```python
from build123d import *

# Parameters (mm, degrees)
F0_W     = 50
F0_H     = 50
F1_DEPTH = 25
F2_R     = 12.5410475497
F3_DEPTH = 25
F5_DEPTH = 25
F7_DEPTH = 50
F9_DEPTH = 25
F10_R    = 5


with BuildPart() as f1:
    # F0 (on Front) → F1 (new body)
    with BuildSketch(Plane.XZ):
        Rectangle(F0_W, F0_H)
    extrude(amount=F1_DEPTH)

    # F2 (on face) → F3 (cut)
    with BuildSketch(Plane.XZ.offset(25)):
        Circle(F2_R)
    extrude(amount=-F3_DEPTH, mode=Mode.SUBTRACT)

    # F4 (on face) → F5 (join)
    with BuildSketch(Plane.XZ.offset(25)):
        with BuildLine():
            Line((-8.8678597656, -8.8678597656), (-25, -25))
            Line((-25, -25), (25, -25))
            Line((25, -25), (25, 25))
            Line((25, 25), (8.8678597656, 8.8678597656))
            ThreePointArc((8.8678597656, 8.8678597656), (11.5864171474, 4.7992511218), (12.5410475497, 0))
            ThreePointArc((12.5410475497, 0), (4.7992511218, -11.5864171474), (-8.8678597656, -8.8678597656))
        make_face()
    extrude(amount=F5_DEPTH)

    # F6 (on face) → F7 (cut)
    with BuildSketch(Plane(origin=(0, 0, 0), x_dir=(0, -1, 0), z_dir=(-0.7071067812, 0, 0.7071067812))):
        Polygon((28.62248093, -26.3251687907), (35.0618112076, -33.3145719446), (44.3344770349, -31.2326499178), (47.1678125847, -22.1613247372), (40.7284823072, -15.1719215833), (31.4558164798, -17.2538436101), align=None)
        Polygon((27.4971282132, 24.391054001), (41.3385996573, 13.714221481), (43.6642721295, 31.0397036374), align=None)
    extrude(amount=-F7_DEPTH, mode=Mode.SUBTRACT)

    # F8 (on face) → F9 (join)
    with BuildSketch(Plane.XZ.offset(25)):
        Polygon((-20.9768815232, 21.2787960948), (-24.3413792657, 11.5523586689), (-16.1306745515, 5.3468967076), (-7.691682224, 11.2381477254), (-10.6868028491, 21.084603052), align=None)
    extrude(amount=F9_DEPTH)

    # F10
    f10_edges = [f1.edges().sort_by_distance(p)[0] for p in [
        (25, 0, 0),
        (0, 0, 25),
        (-25, 0, 0),
        (0, 0, -25),
    ]]
    fillet(f10_edges, radius=F10_R)


solid = f1.part
```
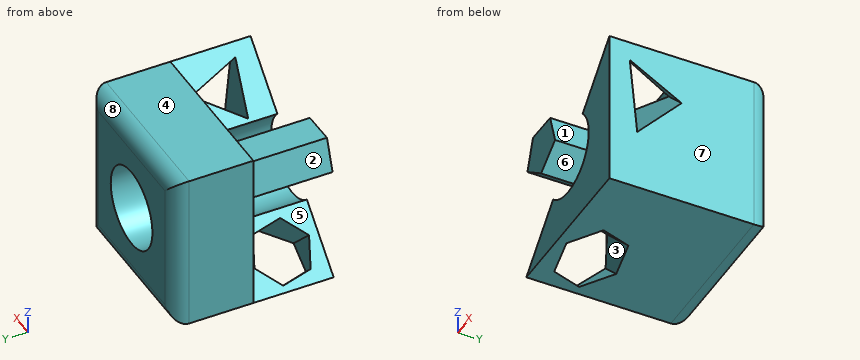
Check sheet for the modelled part. Datum: model origin and axes. Units: mm. Face numbers are marked on the shaded views. A direction names the side the tool comes from. Round coordinates to 2 decimals unless told otherwise and drop trailing zeros. Write each loop counter-clockwise with the first axis right and the second up, starting at its lowest first coordinate (ties: lowest second). Pieces come first, ordered by that corner, then holes. Notation, with made-up numbers: (47, 7.5) -> (90, 7.5) arc R9 ccw to (90, 15.5) -> close; hole circle Ø9 at (35.25, 22). An arc over 180 degrees is marked (long way). One line per question, with ' | ' between items. Start each with the question number.
1. Sectioned sample at C-C, the plane x = 10.5. Record the cut outline in (y, z).
2. Sectioned sample at D-D, the plane y = -39. Record the cut outline in (x, z), then the cut area to 3 significant figures.
3. Depth check by flat-ended pin: pin 1 (1.5 mm diameter, centred on y = -26.5, z = -15, fed in from -X). Enter the tip coordinate at first touch or a pass-through.
4. Release check for a two-part mould opening along Z. For the marked faces 6, 7 and 8 record: +Z half, -Z half, draft (parallel to the pull), parting line (faces both ways), or undercut.
5. Scan lines: line 1 along X through (y, z) = (-17.25, 0); line 2 along Y through (x, z) = (15, 5.5). Record each from-to range of solid material in increasing order. Write a range as from..to.
6. Set-up check for the marked faces 1, 2, 3, 4 and 5: record each of +Z, -Z, +X, -X, +Y, -Y from which the full face is reachable in a straight line by a thin tool's end or side.
7. Sectioned sample at A-A, the plane z = -10. Record the cut outline in (x, y), then the cut area to 3 significant figures.
8. Sectioned sample at B-B, the plane y = -20. Record the cut outline in (x, z), then the cut area to 3 significant figures.
Taken from the geometry:
1) outline: (-50, -25) -> (-5, -25) arc R5 ccw to (0, -20) -> (0, -6.86) -> (-50, -6.86) -> close; (-50, 6.86) -> (0, 6.86) -> (0, 20) arc R5 ccw to (-5, 25) -> (-25, 25) -> (-25, 10.5) -> (-39.87, 10.5) -> (-41.34, 8.89) -> (-41.49, 10.5) -> (-50, 10.5) -> close
2) outline: (-25, -25) -> (-20.86, -25) -> (-22.93, -22.93) -> close; (-24.34, 11.55) -> (-16.13, 5.35) -> (-7.69, 11.24) -> (-10.69, 21.08) -> (-20.98, 21.28) -> close; (-11, -11) -> (2.99, -25) -> (25, -25) -> (25, -3.05) -> (10.97, 10.97) -> (8.87, 8.87) arc R12.54 cw to (-8.87, -8.87) -> close; (20.59, 20.59) -> (25, 16.18) -> (25, 25) -> close | area: 816 mm^2
3) pin 1: stops at x = -15.75
4) face 6: undercut | face 7: draft | face 8: +Z half
5) line 1: x = -25..-12.54, 12.54..25 | line 2: y = -50..-41.44, -40.33..0
6) face 1: +Z, -Y | face 2: +Z, -X, -Y | face 3: none | face 4: +Z, +X, -X, +Y, -Y | face 5: -X, -Y
7) outline: (-25, -25) -> (-10, -25) -> (-10, -50) -> (-7.57, -50) -> (-7.57, 0) -> (-20, 0) arc R5 ccw to (-25, -5) -> close; (7.57, -50) -> (25, -50) -> (25, -5) arc R5 ccw to (20, 0) -> (7.57, 0) -> close | area: 1,360 mm^2
8) outline: (-25, -25) -> (25, -25) -> (25, 25) -> (-25, 25) -> close; hole circle Ø25.08 at (0, 0) | area: 2,010 mm^2
